from build123d import *

# Parameters (mm, degrees)
CHAFL_N1_SIZE2                    = 3.300188603
CHAFL_N1_SIZE                     = 3
CHAFL_N1_EDGE_2_SIZE2             = 3
CHAFL_N1_EDGE_2_SIZE              = 3.300188603
CHAFL_N2_SIZE                     = 0.5
TALADRO_DE_MARGEN_PARA_M101_D     = 11
TALADRO_DE_MARGEN_PARA_M101_DEPTH = 55.695266595
TALADRO_DE_MARGEN_PARA_M101_TIP   = 3.304733405
TALADRO_DE_MARGEN_PARA_M102_D     = 11
TALADRO_DE_MARGEN_PARA_M102_DEPTH = 55.695266595
TALADRO_DE_MARGEN_PARA_M102_TIP   = 3.304733405


with BuildPart() as part:
    # Croquis1 → Revolución1 (revolve)
    with BuildSketch(Plane(origin=(0, 0, 0), x_dir=(0, 0, -1), z_dir=(1, 0, 0))):
        Polygon((0, 0), (0, 12.5), (16.5, 12.5), (20.704376009, 60.556237686), (179.295623991, 60.556237686), (183.5, 12.5), (200, 12.5), (200, 0), align=None)
    revolve(axis=Axis((0, 0, -200), (0, 0, 1)))

    # Chaflán1
    chafl_n1_edges = [part.edges().sort_by_distance(p)[0] for p in [
        (0, -60.556237686, -179.295623991),
    ]]
    chamfer(chafl_n1_edges, length=CHAFL_N1_SIZE, length2=CHAFL_N1_SIZE2)

    # Chaflán1 edge 2
    chafl_n1_edge_2_edges = [part.edges().sort_by_distance(p)[0] for p in [
        (0, -60.556237686, -20.704376009),
    ]]
    chamfer(chafl_n1_edge_2_edges, length=CHAFL_N1_EDGE_2_SIZE, length2=CHAFL_N1_EDGE_2_SIZE2)

    # Chaflán2
    chafl_n2_edges = [part.edges().sort_by_distance(p)[0] for p in [
        (0, -12.5, -200),
        (0, -12.5, 0),
    ]]
    chamfer(chafl_n2_edges, length=CHAFL_N2_SIZE)

    # Taladro de margen para M101
    with Locations(Plane(origin=(0, 0, -200), x_dir=(-1, 0, 0), z_dir=(0, 0, -1))):
        with Locations((0, 0)):
            Hole(TALADRO_DE_MARGEN_PARA_M101_D / 2, depth=TALADRO_DE_MARGEN_PARA_M101_DEPTH)
            with Locations((0, 0, -(TALADRO_DE_MARGEN_PARA_M101_DEPTH + TALADRO_DE_MARGEN_PARA_M101_TIP / 2))):  # 118° drill point
                Cone(0, TALADRO_DE_MARGEN_PARA_M101_D / 2, TALADRO_DE_MARGEN_PARA_M101_TIP, mode=Mode.SUBTRACT)

    # Taladro de margen para M102
    with Locations(Plane.XY):
        with Locations((0, 0)):
            Hole(TALADRO_DE_MARGEN_PARA_M102_D / 2, depth=TALADRO_DE_MARGEN_PARA_M102_DEPTH)
            with Locations((0, 0, -(TALADRO_DE_MARGEN_PARA_M102_DEPTH + TALADRO_DE_MARGEN_PARA_M102_TIP / 2))):  # 118° drill point
                Cone(0, TALADRO_DE_MARGEN_PARA_M102_D / 2, TALADRO_DE_MARGEN_PARA_M102_TIP, mode=Mode.SUBTRACT)


solid = part.part
Check sheet for the modelled part. Datum: model origin and axes. Units: mm. A direction names the side the tool comes from. Coordinates: 2 decimals unless noted, no trailing zeros. Loops run counter-clockwise (first coordinate to the right, second up) from the corner with the lowest first, then second, coordinate; pieces in that order, holes last. Notation, with made-up numbers: (-35, -17) -> (24, -17) arc R17 cw to (24, 7) -> close; hole circle Ø6 at (70, -23.75). An arc over 180 degrees is marked (long way). Answer in a Markdown table with one row per item.
1. Go/stop test with flat-tipped pins: pin 1 (4 mm diameter, centred on x = 15.5, y = 14, fed in from +Z); pin 2 (4 mm diameter, centred on x = 47, z = -89.5, fed in from +Y); pin 3 (1.5 mm diameter, centred on y = -3, z = -62, fed in from +X). Record where each tip stops, or that it passes through.
Check values:
| item | result |
|---|---|
| pin 1 | stops at z = -17.06 |
| pin 2 | stops at y = 40.52 |
| pin 3 | stops at x = 60.51 |
2. Access from +Z, -Z, +X, -X, +Y, -Y to the whole of each face (thin tool, end or side, straight path). Record for faces 1 (the face through (-3.755, 11.923, -8.612)), 2 (the face through (2.5, -5.2, 0)), 3 (the face through (-3.755, 11.923, -191.612)).
Check values:
| item | result |
|---|---|
| face 1 | +Z |
| face 2 | +Z, +X, -X, +Y, -Y |
| face 3 | -Z |
3. Release check for a two-part mould opening along X. For faces 4 (the face through (5.62, 13.55, -183.31)), 5 (the face through (2.5, 5.2, -200)), 6 (the face through (1.19, -5.37, -28.24)) record: released by +X, released by -X, zero draft, split by the parting line, or undercut.
Check values:
| item | result |
|---|---|
| face 4 | split by the parting line |
| face 5 | zero draft |
| face 6 | undercut |
4. Sectioned sample at A-A, the plane z = -152.5. Record the boundary of the cut face in (x, y), then the cut area to 3 significant figures.
Check values:
| item | result |
|---|---|
| outline | circle Ø121.11 at (0, 0); hole circle Ø11 at (0, 0) |
| area | 11,400 mm2 |
5. Material ranges on line 1 along Y through (x, z) = (0, -168); line 2 along Y through (x, z) = (0, -186), recorded low to high. Write a range as [from, to].
Check values:
| item | result |
|---|---|
| line 1 | y = [-60.56, -5.5], [5.5, 60.56] |
| line 2 | y = [-12.5, -5.5], [5.5, 12.5] |
6. Sectioned sample at B-B, the plane z = -114. Record the boundary of the cut face in (x, y).
Check values:
| item | result |
|---|---|
| outline | circle Ø121.11 at (0, 0) |
